```python
from build123d import *

# Parameters (mm, degrees)
BOSS_EXTRUDE1_DEPTH = 27.5844
SKETCH3_R           = 1.6256
CUT_EXTRUDE2_DEPTH  = 16.5575
SKETCH4_R           = 9.525
BOSS_EXTRUDE3_DEPTH = 1.27
SKETCH2_R           = 4.1021
CUT_EXTRUDE1_DEPTH  = 29.8544


with BuildPart() as part:
    # Sketch1 → Boss-Extrude1 (new body)
    with BuildSketch(Plane(origin=(0, 0, 0), x_dir=(1, 0, 0), z_dir=(0, 1, 0))):
        Polygon((-3.592850725, 6.223), (-7.18570145, 0), (-3.592850725, -6.223), (3.592850725, -6.223), (7.18570145, 0), (3.592850725, 6.223), align=None)
    extrude(amount=BOSS_EXTRUDE1_DEPTH)

    # Sketch3 → Cut-Extrude2 (cut, through all)
    with BuildSketch(Plane(origin=(5.389276088, 0, 3.1115), x_dir=(0.5, 0, -0.866025404), z_dir=(0.866025404, 0, 0.5))):
        with Locations((0, 11.2776)):
            Circle(SKETCH3_R)
    extrude(amount=-CUT_EXTRUDE2_DEPTH, mode=Mode.SUBTRACT)

    # Sketch4 → Boss-Extrude3 (add)
    with BuildSketch(Plane.XZ):
        Circle(SKETCH4_R)
    extrude(amount=BOSS_EXTRUDE3_DEPTH)

    # Sketch2 → Cut-Extrude1 (cut, through all)
    with BuildSketch(Plane(origin=(0, 27.5844, 0), x_dir=(1, 0, 0), z_dir=(0, 1, 0))):
        Circle(SKETCH2_R)
    extrude(amount=-CUT_EXTRUDE1_DEPTH, mode=Mode.SUBTRACT)


solid = part.part
```
The model under review builds one solid part; all positions refer to its coordinate system, in mm. A direction names the side the tool comes from. Give positions to 0.01 mm unless a question says otherwise; leave off trailing zeros. Write each loop counter-clockwise with the first axis right and the second up, starting at its lowest first coordinate (ties: lowest second). Pieces come first, ordered by that corner, then holes.
(1) Consider section B-B, the plane y = 4.5. Give the boundary of the cut face in (x, z), and give its area (3 significant figures).
(2) Consider section D-D, the plane z = -2.75. Give the number of separate pieces and of enclosed holes in the cut face, and give its area (3 significant figures).
(3) Consider section C-C, the plane x = -2. Give the boundary of the cut face in (y, z), and give its area (3 significant figures).
(4) The part is to be moulded in two halves that separate along X. For faces 5 (the cylindrical face through (-0.889, 13.359, 4.005)), 6 (the flat face through (1.5, 27.584, -4.2)), 7 (the flat face through (-5.414, 13.599, 3.068)), say which applies: released by +X, released by -X, zero draft, split by the parting line, or undercut.
(5) For P1, Ø8, axis at x = 1.5, y = 11, coming from the -Z side; P2, Ø8, axis at x = 3, y = 18.5, coming from the +Z side; P3, Ø1, axis at x = -3.5, z = 2, coming from the -Y side; P4, Ø1, axis at y = 6, z = 1, coming from the +X side, all flat-tipped, find the tip position at first contact; note any pin that passes through.
(6) To check wall thickness, follow L1, parallel to Z at x = 0, y = 10.75; L2, parallel to Y at x = -6.75, z = 3.75; L3, parallel to X at y = 5.75, z = -3. State the ranges of each line that lie inside material, in increasing order.
(7) Tool access review of faces 1 (the flat face through (6.2, 0, 2.3)), 2 (the flat face through (0, 14, 6.223)), 3 (the flat face through (5.414, 13.599, -3.068)), 4 (the flat face through (0, 14, -6.223)): name each direction out of +Z, -Z, +X, -X, +Y, -Y from which nothing blocks a thin tool from reaching the whole face with its end or side.
(8) Consider section A-A, the plane x = 0. Give the boundary of the cut face in (y, z) (3 decimals), and give its area (3 significant figures).
Returned:
1. outline: (-7.19, 0) - (-3.59, -6.22) - (3.59, -6.22) - (7.19, 0) - (3.59, 6.22) - (-3.59, 6.22) - close; hole circle Ø8.2 at (0, 0)
1. area: 81.3 mm2
2. separate pieces: 3
2. enclosed holes: 0
2. area: 148 mm2
3. outline: (-1.27, -9.31) - (0, -9.31) - (0, -6.22) - (27.58, -6.22) - (27.58, -3.58) - (-1.27, -3.58) - close; (-1.27, 3.58) - (27.58, 3.58) - (27.58, 6.22) - (0, 6.22) - (0, 9.31) - (-1.27, 9.31) - close
3. area: 160 mm2
4. face 5: undercut
4. face 6: zero draft
4. face 7: released by -X
5. P1: stops at z = -6.22
5. P2: stops at z = 6.22
5. P3: stops at y = -1.27
5. P4: stops at x = 6.9
6. L1: z = -6.22 to -4.1, 4.1 to 6.22
6. L2: y = -1.27 to 0
6. L3: x = -5.45 to -2.8, 2.8 to 5.45
7. face 1: +Y
7. face 2: +Z, +X, -X, +Y
7. face 3: -Z, +X, +Y
7. face 4: -Z, +X, -X, +Y
8. outline: (-1.27, -9.525) - (0, -9.525) - (0, -6.223) - (27.584, -6.223) - (27.584, -4.102) - (-1.27, -4.102) - close; (-1.27, 4.102) - (27.584, 4.102) - (27.584, 6.223) - (0, 6.223) - (0, 9.525) - (-1.27, 9.525) - close
8. area: 131 mm2
